from build123d import *

# Parameters (mm, degrees)
F1_DEPTH = 5


with BuildPart() as f1:
    # F0 (on Front) → F1 (new body)
    with BuildSketch(Plane.XZ):
        with BuildLine():
            Line((0, 17.5), (0, 21.5))
            ThreePointArc((0, 21.5), (-20.376797, 6.858291), (-13, -17.124544))
            Line((-13, -17.124544), (-13.567663, -27.956202))
            Line((-13.567663, -27.956202), (-23.567663, -27.956202))
            ThreePointArc((-23.567663, -27.956202), (-32.89779, -30.456202), (-23.567663, -32.956202))
            Line((-23.567663, -32.956202), (-13.829702, -32.956202))
            Line((-13.829702, -32.956202), (-14.907737, -53.526337))
            ThreePointArc((-14.907737, -53.526337), (-22.389872, -63.378031), (-34.302261, -60.041385))
            ThreePointArc((-34.302261, -60.041385), (-36.688307, -56.897738), (-38.739987, -53.526337))
            Line((-38.739987, -53.526337), (-34.511764, -56.051488))
            Line((-34.511764, -56.051488), (-42.037944, -45.259527))
            Line((-42.037944, -45.259527), (-43.209494, -58.364384))
            Line((-43.209494, -58.364384), (-40.79404, -54.07255))
            ThreePointArc((-40.79404, -54.07255), (-35.239888, -63.015457), (-26.595041, -69.023021))
            ThreePointArc((-26.595041, -69.023021), (-16.881661, -74.035451), (-8, -80.406505))
            Line((-8, -80.406505), (-8, -19.956202))
            Line((-8, -19.956202), (-8, -15.564382))
            ThreePointArc((-8, -15.564382), (-17.009214, 4.115417), (0, 17.5))
        make_face()
    extrude(amount=F1_DEPTH)

    # F2: F1 across face


with BuildPart() as f1_1:
    add(f1.part)
    add(f1.part.mirror(Plane(origin=(0, -2.5, 19.5), x_dir=(0, 1, 0), z_dir=(1, 0, 0))))


solid = f1_1.part
The listing builds one solid part. Answer for the finished solid, in the listing's coordinates (mm). A direction names the side the tool comes from. Give positions to 0.01 mm unless a question says otherwise; leave off trailing zeros. Loops run counter-clockwise (first coordinate to the right, second up) from the corner with the lowest first, then second, coordinate; pieces in that order, holes last. Notation, with made-up numbers: (36.25, 72.5) - (46.25, 72.5) arc R22 cw to (46.25, 96.5) - close; hole circle Ø1 at (4.5, 33). An arc over 180 degrees is marked (long way). Answer as a JSON object with one key per item and string values.
1. A cutting plane is placed at B-B (z = -30.5). Write down the section's boundary in (x, y), then the cut area to 3 significant figures.
Determined:
{"outline": "(-32.9, -5) - (-8, -5) - (-8, 0) - (-32.9, 0) - close; (8, -5) - (32.9, -5) - (32.9, 0) - (8, 0) - close", "area": "249 mm²"}
2. Find the intervals of material crossed by L1, parallel to X at y = -3.7, z = -33; L2, parallel to X at y = -4.55, z = -26.5; L3, parallel to X at y = -3.6, z = -58, in increasing order. Write a range as [from, to].
Determined:
{"L1": "[-32.2, -23.59], [-13.83, -8], [8, 13.83], [23.59, 32.2]", "L2": "[-30.96, -24.84], [-13.49, -8], [8, 13.49], [24.84, 30.96]", "L3": "[-43.18, -43], [-38.97, -35.91], [-16.12, -8], [8, 16.12], [35.91, 38.97], [43, 43.18]"}
3. A cutting plane is placed at D-D (x = -3). Write down the section's boundary in (y, z).
Determined:
{"outline": "(-5, 17.24) - (0, 17.24) - (0, 21.29) - (-5, 21.29) - close"}
4. For faces 1 (the flat face through (38.222, -2.465, -50.731)), 2 (the flat face through (8, -2, -48)), 3 (the cylindrical face through (-22.22, -2.46, -63.32)), 4 (the cylindrical face through (17.012, -2.465, -73.956)), determine the directions among +Z, -Z, +X, -X, +Y, -Y from which every point of the face is accessible in a straight line to the end or side of a thin tool.
Determined:
{"face 1": "+Z, +Y, -Y", "face 2": "-Z, +Y, -Y", "face 3": "+Y, -Y", "face 4": "-Z, +X, +Y, -Y"}
5. A cutting plane is placed at A-A (x = 30.5). Write down the section's boundary in (y, z), then the cut area to 3 significant figures.
Determined:
{"outline": "(-5, -66.95) - (0, -66.95) - (0, -62.94) - (-5, -62.94) - close; (-5, -34.73) - (0, -34.73) - (0, -26.19) - (-5, -26.19) - close", "area": "62.7 mm²"}
6. For a pull along X with two mould halves and no side action, classify faces 5 (the flat face through (42.02, -2.46, -56.25)), 6 (the flat face through (-42.616, -2.465, -51.72)), 7 (the flat face through (-9, 0, -37)) as pulls with the +X half, pulls with the -X half, needs draft (parallel to the pull), parting line crosses it, or undercut.
Determined:
{"face 5": "undercut", "face 6": "pulls with the -X half", "face 7": "needs draft"}
7. Flat-ended cylindrical pins translate along their axes: pin 1 Ø2.5 at (y, z) = (-3, -45.5) entering from +X; pin 2 Ø2 at (x, y) = (8.5, -4) entering from +Z; pin 3 Ø1 at (x, y) = (-13, -0.5) entering from +Z. Find the tip coordinate at first contact, or state that the pin passes through.
Determined:
{"pin 1": "x = 42.17", "pin 2": "z = 20.15", "pin 3": "z = 17.49"}
